```python
from build123d import *

# Parameters (mm, degrees)
BOSS_EXTRU_3_DEPTH      = 30
ESQUISSE1_5_W           = 12.875644347
ESQUISSE1_5_H           = 12
BOSS_EXTRU_4_DEPTH      = 30
ESQUISSE10_R            = 1.5
ENL_V_MAT_EXTRU_1_DEPTH = 3
ESQUISSE9_R             = 1.5
ENL_V_MAT_EXTRU_2_DEPTH = 3
ESQUISSE11_R            = 2
ENL_V_MAT_EXTRU_3_DEPTH = 13


with BuildPart() as part:
    # Esquisse1 → Boss.-Extru.3 (new body)
    with BuildSketch(Plane(origin=(0, 0, 0), x_dir=(1, 0, 0), z_dir=(0, 1, 0))):
        with BuildLine():
            Line((-12.124355653, 7), (-12.124355653, 19))
            Line((-12.124355653, 19), (12.124355653, 19))
            Line((12.124355653, 19), (12.124355653, 7))
            ThreePointArc((12.124355653, 7), (0, 14), (-12.124355653, 7))
        make_face()
    extrude(amount=BOSS_EXTRU_3_DEPTH)

    # Esquisse1_5 → Boss.-Extru.4 (add)
    with BuildSketch(Plane(origin=(0, 0, 0), x_dir=(1, 0, 0), z_dir=(0, 1, 0))):
        with Locations((-18.562177827, 13)):
            Rectangle(ESQUISSE1_5_W, ESQUISSE1_5_H)
        with Locations((18.562177827, 13)):
            Rectangle(ESQUISSE1_5_W, ESQUISSE1_5_H)
    extrude(amount=BOSS_EXTRU_4_DEPTH)

    # Esquisse10 → Enl_v. mat.-Extru.1 (cut)
    with BuildSketch(Plane(origin=(25, 0, 0), x_dir=(0, 0, -1), z_dir=(1, 0, 0))):
        with Locations((13, 25)):
            Circle(ESQUISSE10_R)
        with Locations((13, 5)):
            Circle(ESQUISSE10_R)
    extrude(amount=-ENL_V_MAT_EXTRU_1_DEPTH, mode=Mode.SUBTRACT)

    # Esquisse9 → Enl_v. mat.-Extru.2 (cut)
    with BuildSketch(Plane.ZY.offset(25)):
        with Locations((-13, 25)):
            Circle(ESQUISSE9_R)
        with Locations((-13, 5)):
            Circle(ESQUISSE9_R)
    extrude(amount=-ENL_V_MAT_EXTRU_2_DEPTH, mode=Mode.SUBTRACT)

    # Esquisse11 → Enl_v. mat.-Extru.3 (cut, through all)
    with BuildSketch(Plane(origin=(0, 0, -19), x_dir=(-1, 0, 0), z_dir=(0, 0, -1))):
        with Locations((-20, 20)):
            Circle(ESQUISSE11_R)
        with Locations((20, 20)):
            Circle(ESQUISSE11_R)
        with Locations((-20, 10)):
            Circle(ESQUISSE11_R)
        with Locations((20, 10)):
            Circle(ESQUISSE11_R)
    extrude(amount=-ENL_V_MAT_EXTRU_3_DEPTH, mode=Mode.SUBTRACT)


solid = part.part
```
The model under review builds one solid part; all positions refer to its coordinate system, in mm. A direction names the side the tool comes from. Give positions to 0.01 mm unless a question says otherwise; leave off trailing zeros. Write each loop counter-clockwise with the first axis right and the second up, starting at its lowest first coordinate (ties: lowest second). Pieces come first, ordered by that corner, then holes.
(1) Consider section D-D, the plane z = -16.5. Give the boundary of the cut face in (x, y).
(2) Consider section C-C, the plane z = -10.75. Give the boundary of the cut face in (x, y), and give its area (3 significant figures).
(3) The part is to be moulded in two halves that separate along X. For faces 4 (the flat face through (-22, 25, -13)), 5 (the flat face through (22, 5, -13)), 6 (the cylindrical face through (-18.526, 11.352, -13.084)), say which applies: released by +X, released by -X, zero draft, split by the parting line, or undercut.
(4) For P1, Ø1.5, axis at y = 25, z = -12.5, coming from the +X side; P2, Ø3.5, axis at y = 5, z = -12.5, coming from the +X side; P3, Ø1.8, axis at y = 25, z = -13, coming from the -X side, all flat-tipped, find the tip position at first contact; note any pin that passes through.
(5) Consider section A-A, the plane x = 20. Give the boundary of the cut face in (y, z), and give its area (3 significant figures).
(6) To check wall thickness, follow L1, parallel to Y at x = 20, z = -11.25; L2, parallel to Y at x = 24.3, z = -13; L3, parallel to X at y = 19.75, z = -10. State the ranges of each line that lie inside material, in increasing order.
(7) Consider section B-B, the plane y = 20. Give the boundary of the cut face in (x, z).
(8) Tool access review of faces 1 (the cylindrical face through (-23.52, 5.07, -14.5)), 2 (the flat face through (0, 15, -19)), 3 (the cylindrical face through (23.52, 5.07, -11.5)): name each direction out of +Z, -Z, +X, -X, +Y, -Y from which nothing blocks a thin tool from reaching the whole face with its end or side.
Returned:
1. outline: (-25, 0) - (25, 0) - (25, 30) - (-25, 30) - close; hole circle Ø4 at (-20, 10); hole circle Ø4 at (-20, 20); hole circle Ø4 at (20, 10); hole circle Ø4 at (20, 20)
2. outline: (-25, 0) - (-8.97, 0) - (-8.97, 30) - (-25, 30) - close; (8.97, 0) - (25, 0) - (25, 30) - (8.97, 30) - close; hole circle Ø4 at (-20, 10); hole circle Ø4 at (-20, 20); hole circle Ø4 at (20, 10); hole circle Ø4 at (20, 20)
2. area: 912 mm2
3. face 4: released by -X
3. face 5: released by +X
3. face 6: undercut
4. P1: stops at x = 22
4. P2: stops at x = 25
4. P3: stops at x = -22
5. outline: (0, -19) - (8, -19) - (8, -7) - (0, -7) - close; (12, -19) - (18, -19) - (18, -7) - (12, -7) - close; (22, -19) - (30, -19) - (30, -7) - (22, -7) - close
5. area: 264 mm2
6. L1: y = 0 to 8, 12 to 18, 22 to 30
6. L2: y = 0 to 3.5, 6.5 to 23.5, 26.5 to 30
6. L3: x = -25 to -21.98, -18.02 to -9.8, 9.8 to 18.02, 21.98 to 25
7. outline: (-25, -19) - (-22, -19) - (-22, -7) - (-25, -7) - close; (-18, -19) - (18, -19) - (18, -7) - (12.12, -7) arc R14 cw to (-12.12, -7) - (-18, -7) - close; (22, -19) - (25, -19) - (25, -7) - (22, -7) - close
8. face 1: -X
8. face 2: -Z, +X, -X, +Y, -Y
8. face 3: +X
